from build123d import *

# Parameters (mm, degrees)
F1_DEPTH = 27
F0_W     = 6.4
F0_H     = 19.8
F0_R     = 2.5
F2_DEPTH = 2.54
F3_R     = 5.08
F5_D     = 3.81
F6_R     = 1.27


with BuildPart() as f1:
    # F0 (on Top) → F1 (new body)
    with BuildSketch(Plane.XY):
        Polygon((36.7, 1.27), (26.7, 1.27), (-26.7, 1.27), (-36.7, 1.27), (-36.7, -1.27), (-26.7, -1.27), (-20.3, -1.27), (20.3, -1.27), (26.7, -1.27), (36.7, -1.27), align=None)
    extrude(amount=-F1_DEPTH)

    # F0 (on Top) → F2 (join)
    with BuildSketch(Plane.XY):
        with Locations((-23.5, -11.17)):
            Rectangle(F0_W, F0_H)
        with Locations((-23.5, -16.17)):
            Circle(F0_R, mode=Mode.SUBTRACT)
        with Locations((-23.5, -6.17)):
            Circle(F0_R, mode=Mode.SUBTRACT)
        with Locations((23.5, -11.17)):
            Rectangle(F0_W, F0_H)
        with Locations((23.5, -16.17)):
            Circle(F0_R, mode=Mode.SUBTRACT)
        with Locations((23.5, -6.17)):
            Circle(F0_R, mode=Mode.SUBTRACT)
    extrude(amount=-F2_DEPTH)

    # F3
    f3_edges = [f1.edges().sort_by_distance(p)[0] for p in [
        (-36.7, 0, 0),
        (36.7, 0, 0),
        (36.7, 0, -27),
        (-36.7, 0, -27),
    ]]
    fillet(f3_edges, radius=F3_R)

    # F5 (through all)
    with Locations(Plane.XZ.offset(1.27)):
        with Locations((-30.41523, -3.90541), (-30.41523, -23.09459), (30.41523, -3.90541), (30.41523, -23.09459)):
            Hole(F5_D / 2)

    # F6
    f6_edges = [f1.edges().sort_by_distance(p)[0] for p in [
        (-20.3, -21.07, -1.27),
        (-26.7, -21.07, -1.27),
        (20.3, -21.07, -1.27),
        (26.7, -21.07, -1.27),
    ]]
    fillet(f6_edges, radius=F6_R)


solid = f1.part
Check sheet for the modelled part. Datum: model origin and axes. Units: mm. A direction names the side the tool comes from. Give positions to 0.01 mm unless a question says otherwise; leave off trailing zeros. Write each loop counter-clockwise with the first axis right and the second up, starting at its lowest first coordinate (ties: lowest second). Pieces come first, ordered by that corner, then holes. Notation, with made-up numbers: M 28,69 L 66,69 A22 cw 66,107 Z; hole C -9,29 d6. An arc over 180 degrees is marked long. Use one line per item in the form item = value.
(1) Tool access check on faces 4 (the flat face through (-24, -11, -2.54)), 5 (the flat face through (-26.7, -11, -1)), 6 (the cylindrical face through (20.682, -20.708, -1.288)), 7 (the cylindrical face through (-25.34, -14.48, -1.25)). Record the directions out of +Z, -Z, +X, -X, +Y, -Y that give a thin tool (end or side, any length) a straight path to the whole face; none if there is none.
Answer block:
face_4 = -Z, +X, -X, -Y
face_5 = +Z, -Z, -X, -Y
face_6 = +Z, -Z, -Y
face_7 = +Z, -Z
(2) Depth check by flat-ended pin: P1, Ø1.3, axis at y = -8.5, z = -1.5, coming from the -X side; P2, Ø8, axis at x = 23.5, y = -6.17, coming from the -Z side; P3, Ø1.3, axis at y = -7, z = -1, coming from the +X side. Enter the tip coordinate at first touch or a pass-through.
Answer block:
P1 = -26.7
P2 = -2.54
P3 = 26.7
(3) Section check A-A on y = -11.5. Record the boundary of the cut face in (x, z), plus the area to 3 significant figures.
Answer block:
outline = M -26.7,-2.54 L -20.3,-2.54 L -20.3,0 L -26.7,0 Z; M 20.3,-2.54 L 26.7,-2.54 L 26.7,0 L 20.3,0 Z
area = 32.5 mm2
(4) Section check C-C on y = -16.17. Record the boundary of the cut face in (x, z).
Answer block:
outline = M -26.7,-2.54 L -26,-2.54 L -26,0 L -26.7,0 Z; M -21,-2.54 L -20.3,-2.54 L -20.3,0 L -21,0 Z; M 20.3,-2.54 L 21,-2.54 L 21,0 L 20.3,0 Z; M 26,-2.54 L 26.7,-2.54 L 26.7,0 L 26,0 Z
(5) Section check B-B on x = -23.5. Record the boundary of the cut face in (y, z).
Answer block:
outline = M -21.07,-2.54 L -18.67,-2.54 L -18.67,0 L -21.07,0 Z; M -13.67,-2.54 L -8.67,-2.54 L -8.67,0 L -13.67,0 Z; M -3.67,-2.54 L -1.27,-2.54 L -1.27,-27 L 1.27,-27 L 1.27,0 L -3.67,0 Z
(6) Material ranges on line 1 along Y through (x, z) = (23.5, -0.65); line 2 along X through (y, z) = (-0.5, -5); line 3 along Y through (x, z) = (1.5, -17.75), recorded low to high.
Answer block:
line_1 = -21.07 to -18.67, -13.67 to -8.67, -3.67 to 1.27
line_2 = -36.7 to -31.97, -28.86 to 28.86, 31.97 to 36.7
line_3 = -1.27 to 1.27
(7) Section check D-D on z = -19.75. Record the boundary of the cut face in (x, y).
Answer block:
outline = M -36.7,-1.27 L 36.7,-1.27 L 36.7,1.27 L -36.7,1.27 Z
(8) Draft check along Z on faces 1 (the cylindrical face through (-28.9, 0.02, -24.25)), 2 (the flat face through (0, 0, -27)), 3 (the flat face through (-1, -1.27, -13)). Enter one of: pulls with the +Z half, pulls with the -Z half, needs draft (parallel to the pull), parting line crosses it, or undercut.
Answer block:
face_1 = undercut
face_2 = pulls with the -Z half
face_3 = needs draft
